Geometry check sheet. Reference: the model listing, model coordinates, mm. A direction names the side the tool comes from. Give positions to 0.01 mm unless a question says otherwise; leave off trailing zeros. Order: outer loops, then holes, each group sorted by start corner. A loop starts at its lowest first (then second) coordinate and runs counter-clockwise, first axis right, second up.
Autodesk Inventor part; units mm, degrees
ref_plane "Work Plane1" through (0, 8, 0) normal (0, 1, 0) x (1, 0, 0)
ref_plane "YZ Plane" through (0, 0, 0) normal (1, 0, 0) x (0, 1, 0)
ref_plane "XZ Plane" through (0, 0, 0) normal (0, 1, 0) x (-1, 0, 0)
sketch "Sketch1" plane through (0, 0, 0) normal (0, 1, 0) x (-1, 0, 0)
  arc A0 (31.569, 13.7227) -> (30.069, 12.2227) centre (31.569, 12.2227) ccw
  line L0 (31.569, 13.7227) -> (34.069, 13.7227)
  line L1 (34.069, 13.7227) -> (34.069, 18.9227)
  line L2 (32.069, 20.9227) -> (0.569, 20.9227)
  line L3 (-1.431, -13.7773) -> (0.569, -13.7773)
  line L4 (0.569, -13.7773) -> (0.569, -18.2773)
  line L5 (34.069, -13.2773) -> (31.569, -13.2773)
  arc A1 (30.069, -11.7773) -> (31.569, -13.2773) centre (31.569, -11.7773) ccw
  arc A2 (34.069, 18.9227) -> (32.069, 20.9227) centre (32.069, 18.9227) ccw
  arc A3 (34.0195, 22.4149) -> (32.069, 23.9727) centre (32.069, 21.9727) ccw
  line L6 (32.069, 23.9727) -> (-23.931, 23.9727)
  arc A4 (-23.931, 23.9727) -> (-25.931, 21.9727) centre (-23.931, 21.9727) ccw
  line L7 (-25.931, 21.9727) -> (-25.931, -21.0273)
  arc A5 (-25.931, -21.0273) -> (-23.931, -23.0273) centre (-23.931, -21.0273) ccw
  line L8 (-23.931, -23.0273) -> (32.069, -23.0273)
  arc A6 (32.069, -23.0273) -> (33.899, -21.8341) centre (32.069, -21.0273) ccw
  arc A7 (32.069, -20.2773) -> (34.069, -18.2773) centre (32.069, -18.2773) ccw
  line L9 (32.069, -20.2773) -> (2.569, -20.2773)
  arc A8 (0.569, -18.2773) -> (2.569, -20.2773) centre (2.569, -18.2773) ccw
  line L10 (34.069, -13.2773) -> (34.069, 13.7227)
  line L11 (0.569, -13.7773) -> (0.569, 20.9227)
  line L12 (30.069, -11.7773) -> (30.069, 12.2227)
  line L13 (0.569, 22.9227) -> (0.569, 20.9227)
  line L14 (34.069, -18.2773) -> (34.069, -13.2773)
  line L15 (0.569, 22.9227) -> (32.069, 22.9227)
  arc A9 (36.069, 18.9227) -> (32.069, 22.9227) centre (32.069, 18.9227) ccw
  line L16 (-1.431, -13.7773) -> (-1.431, -18.2773)
  arc A10 (-1.431, -18.2773) -> (2.569, -22.2773) centre (2.569, -18.2773) ccw
  line L17 (2.569, -22.2773) -> (32.069, -22.2773)
  arc A11 (32.069, -22.2773) -> (36.069, -18.2773) centre (32.069, -18.2773) ccw
  line L18 (36.069, -18.2773) -> (36.069, 18.9227)
  dimension "d8" = 2
  dimension "d9" = 2
extrude "Extrusion3" add sketch "Sketch1" against normal blind 2 contours L0 L10 L5 A1 L12 A0 | A0 L12 A1 L5 L14 A7 L9 A8 L4 L11 L2 A2 L1 L0 | L1 A2 L2 L13 L15 A9 L18 A11 L17 A10 L16 L3 L4 A8 L9 A7 L14 L10
ref_plane "Work Plane1" through (0, 8, 0) normal (0, 1, 0) x (1, 0, 0)
extrude "Extrusion4" add sketch "Sketch1" along normal blind 8 contours L1 A2 L2 L13 L15 A9 L18 A11 L17 A10 L16 L3 L4 A8 L9 A7 L14 L10
sketch "Sketch2" plane through (0, 8, 0) normal (0, 1, 0) x (1, 0, 0)
  line L0 (23.931, 23.0273) -> (-32.069, 23.0273)
  arc A0 (-32.069, 23.0273) -> (-33.899, 21.8341) centre (-32.069, 21.0273) ccw
  line L1 (-32.069, -23.9727) -> (23.931, -23.9727)
  arc A1 (-34.0195, -22.4149) -> (-32.069, -23.9727) centre (-32.069, -21.9727) ccw
  line L2 (-36.069, 18.2773) -> (-36.069, -18.9227)
  arc A2 (-32.069, 23.0273) -> (-34.069, 21.0273) centre (-32.069, 21.0273) ccw
  arc A3 (-34.069, -21.9727) -> (-32.069, -23.9727) centre (-32.069, -21.9727) ccw
  line L3 (-34.069, 18.2773) -> (-34.069, 13.2773)
  line L4 (-34.069, 13.2773) -> (-34.069, -13.7227)
  line L5 (-34.069, -13.7227) -> (-34.069, -18.9227)
  line L6 (-34.069, -21.9727) -> (-34.069, 21.0273)
  arc A4 (-32.069, 25.0273) -> (-36.069, 21.0273) centre (-32.069, 21.0273) ccw
  line L7 (-36.069, 21.0273) -> (-36.069, -21.9727)
  arc A5 (-36.069, -21.9727) -> (-32.069, -25.9727) centre (-32.069, -21.9727) ccw
  line L8 (-0.569, 25.0273) -> (-32.069, 25.0273)
  arc A6 (-32.069, 25.0273) -> (-35.729, 22.6409) centre (-32.069, 21.0273) ccw
  line L9 (-0.569, -25.9727) -> (-32.069, -25.9727)
  arc A7 (-35.97, -22.8571) -> (-32.069, -25.9727) centre (-32.069, -21.9727) ccw
  line L10 (-0.569, 13.7773) -> (-0.569, -22.9227)
  line L11 (-0.569, -23.9727) -> (-0.569, -25.9727)
  line L12 (-0.569, 18.2773) -> (-0.569, 25.0273)
  line L13 (-0.569, 13.7773) -> (-0.569, 18.2773)
  line L14 (-32.069, 23.0273) -> (-0.569, 23.0273)
  line L15 (-32.069, -23.9727) -> (-0.569, -23.9727)
  arc A8 (-0.569, 18.2773) -> (-2.569, 20.2773) centre (-2.569, 18.2773) ccw
  line L16 (-32.069, -20.9227) -> (-0.569, -20.9227)
  line L17 (-0.569, -20.9227) -> (-0.569, 13.7773)
  line L18 (-0.569, 13.7773) -> (-0.569, 18.2773)
  arc A9 (-0.569, 18.2773) -> (-2.569, 20.2773) centre (-2.569, 18.2773) ccw
  line L19 (-2.569, 20.2773) -> (-32.069, 20.2773)
  arc A10 (-32.069, 20.2773) -> (-34.069, 18.2773) centre (-32.069, 18.2773) ccw
  line L20 (-34.069, 18.2773) -> (-34.069, -18.9227)
  arc A11 (-34.069, -18.9227) -> (-32.069, -20.9227) centre (-32.069, -18.9227) ccw
  line L21 (-0.569, -23.9727) -> (-0.569, -22.9227)
  line L22 (-32.069, 22.2773) -> (-2.569, 22.2773)
  line L23 (-2.569, 22.2773) -> (-0.569, 22.2773)
  arc A12 (1.431, 18.2773) -> (-2.569, 22.2773) centre (-2.569, 18.2773) ccw
  point P0 (0, 0)
  point P1 (-0.569, 21.7414)
  dimension "d18" = 2
  dimension "d19" = 2
  dimension "d20" = 2
  dimension "d21" = 31.5
  dimension "d22" = 31.5
  dimension "d23" = 31.5
sketch "Sketch3" plane through (0, 8, 0) normal (0, 1, 0) x (1, 0, 0)
  line L0 (-0.569, 18.2773) -> (-0.569, 13.7773)
  line L1 (-0.569, 13.7773) -> (1.431, 13.7773)
  line L2 (1.431, 13.7773) -> (1.431, 18.2773)
  arc A0 (1.431, 18.2773) -> (-2.569, 22.2773) centre (-2.569, 18.2773) ccw
  line L3 (-0.569, -20.9227) -> (-32.069, -20.9227)
  arc A1 (-34.069, -18.9227) -> (-32.069, -20.9227) centre (-32.069, -18.9227) ccw
  line L4 (-34.069, -18.9227) -> (-34.069, 18.2773)
  arc A2 (-32.069, 20.2773) -> (-34.069, 18.2773) centre (-32.069, 18.2773) ccw
  line L5 (-32.069, 20.2773) -> (-2.569, 20.2773)
  arc A3 (-0.569, 18.2773) -> (-2.569, 20.2773) centre (-2.569, 18.2773) ccw
  arc A4 (-32.069, 22.2773) -> (-36.069, 18.2773) centre (-32.069, 18.2773) ccw
  line L6 (-36.069, 18.2773) -> (-36.069, -18.9227)
  arc A5 (-36.069, -18.9227) -> (-32.069, -22.9227) centre (-32.069, -18.9227) ccw
  line L7 (-32.069, -22.9227) -> (-0.569, -22.9227)
  line L8 (-0.569, -22.9227) -> (-0.569, -20.9227)
  line L9 (-2.569, 22.2773) -> (-32.069, 22.2773)
  point P0 (0, 0)
extrude "Extrusion7" add sketch "Sketch2" against normal blind 2 contours L12 L23 A12 A8 L19 A10 L6 A2 A0 L0 | L0 A0 A2 L6 L3 L4 L5 A3 A1 L1 L11 L9 A5 L7 L2 A4 L8 L12 | L12 A12 L23 | L10 L21 L1 A1 A3 L6 A11 L16
extrude "Extrusion8" add sketch "Sketch2" along normal blind 15 contours L0 A0 A2 L6 L3 L4 L5 A3 A1 L1 L11 L9 A5 L7 L2 A4 L8 L12
sketch "Sketch4" plane through (0, 8, 0) normal (0, 1, 0) x (1, 0, 0)
  line L0 (1.431, 13.7773) -> (1.431, 18.2773)
  line L1 (-0.569, 13.7773) -> (1.431, 13.7773)
  line L2 (-0.569, 18.2773) -> (-0.569, 25.0273)
  line L3 (-0.569, 18.2773) -> (-0.569, 13.7773)
  arc A0 (1.431, 18.2773) -> (-0.569, 21.7414) centre (-2.569, 18.2773) ccw
  point P0 (0, 0)
extrude "Extrusion9" cut sketch "Sketch4" against normal blind 6
sketch "Sketch5" plane through (0, 23, 0) normal (0, 1, 0) x (1, 0, 0)
  circle A0 centre (-17.319, 30.0273) radius 5
  circle A1 centre (-17.319, 30.0273) radius 3
  line L0 (-0.569, 25.0273) -> (-32.069, 25.0273)
  arc A2 (-12.4777, 28.7773) -> (-9.573, 25.0273) centre (-9.573, 28.0273) ccw
  arc A3 (-25.0649, 25.0273) -> (-22.1602, 28.7773) centre (-25.0649, 28.0273) ccw
  line L1 (-0.569, 23.0273) -> (-0.569, 25.0273)
  line L2 (-34.069, -21.9727) -> (-34.069, 21.0273)
  circle A4 centre (-6.0917, -30.9727) radius 5
  circle A5 centre (-6.0917, -30.9727) radius 2.5
  arc A6 (-10.305, -28.2804) -> (-11.569, -25.9727) centre (-11.569, -27.4727) ccw
  arc A7 (-0.6145, -25.9727) -> (-1.8785, -28.2804) centre (-0.6145, -27.4727) ccw
  line L3 (-32.069, -25.9727) -> (-0.569, -25.9727)
  circle A8 centre (-26.5917, -30.9727) radius 5
  circle A9 centre (-26.5917, -30.9727) radius 2.5
  arc A10 (-30.805, -28.2804) -> (-32.069, -25.9727) centre (-32.069, -27.4727) ccw
  arc A11 (-21.1145, -25.9727) -> (-22.3785, -28.2804) centre (-21.1145, -27.4727) ccw
  line L4 (-0.569, -25.9727) -> (-0.569, -23.9727)
  arc A12 (-36.069, -21.9727) -> (-32.069, -25.9727) centre (-32.069, -21.9727) ccw
  point P0 (0, 0)
  point P1 (1.0185, -24.3852)
  dimension "d34" = 10
  dimension "d35" = 6
  dimension "d36" = 33.5
  dimension "d37" = 16.75
  dimension "d38" = 3
  dimension "d39" = 3
  dimension "d40" = 10
  dimension "d41" = 5
  dimension "d42" = 3
  dimension "d43" = 3
  dimension "d44" = 10
  dimension "d45" = 5
  dimension "d46" = 3
  dimension "d47" = 3
  dimension "d49" = 20.5
extrude "Extrusion10" add sketch "Sketch5" against normal blind 2
sketch "Sketch6" plane through (0, -2, 0) normal (0, -1, 0) x (1, 0, 0)
  line L0 (1.431, -18.2773) -> (1.431, -13.7773)
  line L1 (1.431, -13.7773) -> (-0.569, -13.7773)
  line L2 (-0.569, -13.7773) -> (-0.569, 22.9227)
  line L3 (-0.569, 22.9227) -> (-32.069, 22.9227)
  arc A0 (-32.069, 22.9227) -> (-36.069, 18.9227) centre (-32.069, 18.9227) ccw
  line L4 (-36.069, 18.9227) -> (-36.069, -18.2773)
  arc A1 (-36.069, -18.2773) -> (-32.069, -22.2773) centre (-32.069, -18.2773) ccw
  line L5 (-32.069, -22.2773) -> (-2.569, -22.2773)
  arc A2 (-2.569, -22.2773) -> (1.431, -18.2773) centre (-2.569, -18.2773) ccw
  line L6 (-30.069, 18.9227) -> (-6.569, 18.9227)
  line L7 (-4.569, 16.9227) -> (-4.569, -16.2773)
  line L8 (-6.569, -18.2773) -> (-30.069, -18.2773)
  line L9 (-32.069, -16.2773) -> (-32.069, 16.9227)
  arc A3 (-6.569, -18.2773) -> (-4.569, -16.2773) centre (-6.569, -16.2773) ccw
  arc A4 (-32.069, -16.2773) -> (-30.069, -18.2773) centre (-30.069, -16.2773) ccw
  arc A5 (-30.069, 18.9227) -> (-32.069, 16.9227) centre (-30.069, 16.9227) ccw
  arc A6 (-4.569, 16.9227) -> (-6.569, 18.9227) centre (-6.569, 16.9227) ccw
  point P0 (0, 0)
  point P1 (-4.569, 18.9227)
  point P2 (-4.569, -18.2773)
  dimension "d52" = 4
  dimension "d53" = 37.2
  dimension "d54" = 27.5
  dimension "d55" = 4
  dimension "d56" = 2
extrude "Extrusion11" cut sketch "Sketch6" against normal blind 2 contours L6 A6 L7 A3 L8 A4 L9 A5
equation "\"d37\" = 0.5 * d36"
properties part number "CO-1-01-motorControllersMount"
Item 1: Sectioned sample at D-D (y = 14.75). Enter the section's corners in (x, z).
Reported:
outline: (-36.07, -21.03) arc R4 ccw to (-32.07, -25.03) - (-0.57, -25.03) - (-0.57, -23.03) - (-32.07, -23.03) arc R2 cw to (-33.9, -21.83) arc R2 cw to (-34.07, -21.03) - (-34.07, 21.97) arc R2 cw to (-34.02, 22.41) arc R2 cw to (-32.07, 23.97) - (-0.57, 23.97) - (-0.57, 25.97) - (-32.07, 25.97) arc R4 ccw to (-36.07, 21.97) - close
Item 2: Scan lines: L1, parallel to Z at x = -6.5, y = 5; L2, parallel to Z at x = -3.5, y = 20.25; L3, parallel to Y at x = -2, z = 22. Record each from-to range of solid material in increasing order.
Reported:
L1: z = -22.28 to -20.28, 20.92 to 22.92
L2: z = -25.03 to -23.03, 23.97 to 25.97
L3: y = -2 to 8
Item 3: Gauge pin test, flat ends, axial feed: pin 1 (5.5 mm diameter, centred on x = -19, z = 22, fed in from +Y); pin 2 (3 mm diameter, centred on y = 17, z = 19, fed in from +X); pin 3 (2 mm diameter, centred on x = 0, y = 0.5, fed in from +Z); pin 4 (0.6 mm diameter, centred on y = -0.5, z = 3, fed in from +X). Record the tip position at first contact, or that the pin passes through.
Reported:
pin 1: stops at y = 23
pin 2: stops at x = -34.07
pin 3: stops at z = 22.92
pin 4: stops at x = -0.57
Item 4: Sectioned sample at B-B (z = 12). Enter the section's corners in (x, y), and give its area (3 significant figures).
Reported:
outline: (-36.07, -2) - (-32.07, -2) - (-32.07, 0) - (-34.07, 0) - (-34.07, 23) - (-36.07, 23) - close; (-4.57, -2) - (-0.57, -2) - (-0.57, 0) - (-4.57, 0) - close
area: 62.0 mm2
Item 5: Sectioned sample at C-C (x = -19.5). Enter the section's corners in (y, z), and give its area (3 significant figures).
Reported:
outline: (-2, -22.28) - (6, -22.28) - (6, -25.03) - (21, -25.03) - (21, -27.97) - (23, -27.97) - (23, -23.03) - (8, -23.03) - (8, -20.28) - (0, -20.28) - (0, -18.28) - (-2, -18.28) - close; (-2, 18.92) - (0, 18.92) - (0, 20.92) - (8, 20.92) - (8, 23.97) - (23, 23.97) - (23, 25.97) - (6, 25.97) - (6, 22.92) - (-2, 22.92) - close; (21, -34.53) - (23, -34.53) - (23, -32.09) - (21, -32.09) - close
area: 130 mm2
Item 6: Sectioned sample at A-A (y = 3). Enter the section's corners in (x, z), and give its area (3 significant figures).
Reported:
outline: (-36.07, -18.28) arc R4 ccw to (-32.07, -22.28) - (-2.57, -22.28) arc R4 ccw to (-0.57, -21.74) - (-0.57, -18.28) arc R2 cw to (-2.57, -20.28) - (-32.07, -20.28) arc R2 cw to (-34.07, -18.28) - (-34.07, 18.92) arc R2 cw to (-32.07, 20.92) - (-0.57, 20.92) - (-0.57, 22.92) - (-32.07, 22.92) arc R4 ccw to (-36.07, 18.92) - close
area: 220 mm2
Item 7: Draft check along X on faces 6 (the flat face through (-0.569, 1, -16)), 7 (the flat face through (-0.569, 10, -24)), 8 (the flat face through (-16, 15, -23.027)), 9 (the cylindrical face through (-17.191, 22.014, -35.026)). Enter one of: released by +X, released by -X, zero draft, split by the parting line, or undercut.
Reported:
face 6: undercut
face 7: released by +X
face 8: zero draft
face 9: split by the parting line
Item 8: Set-up check for faces 1 (the flat face through (-17.4, 21, -26.8)), 2 (the flat face through (-24, 21, 30)), 3 (the cylindrical face through (-5.14, -1.01, 18.32)), 4 (the flat face through (-17, 8, 23)), 5 (the flat face through (-18, 4, -20.277)): record each of +Z, -Z, +X, -X, +Y, -Y from which the full face is reachable in a straight line by a thin tool's end or side.
Reported:
face 1: -Z, +X, -X, -Y
face 2: +Z, +X, -X, -Y
face 3: +Y, -Y
face 4: +X, +Y
face 5: +Y
